```python
from build123d import *

# Parameters (mm, degrees)
SKETCH_1_R                    = 85
EXTRUDE_1_DEPTH               = 50
HOLE_WIZARD_M12_1_D           = 13
HOLE_WIZARD_M12_1_CBORE_D     = 22
HOLE_WIZARD_M12_1_CBORE_DEPTH = 15
PATTERN_CIRCULAR_1_COUNT      = 8
SKETCH_6_W                    = 44.766058572
SKETCH_6_H                    = 9.083836387
SKETCH_6_H_2                  = 8.147377862
CUT_EXTRUDE_1_DEPTH           = 131.192165663
SKETCH_7_R                    = 16
CUT_EXTRUDE_2_DEPTH           = 20
SKETCH_8_R                    = 9
CUT_EXTRUDE_3_DEPTH           = 175.530799574
CHAMFER_1_SIZE                = 2
SKETCH_9_R                    = 55
EXTRUDE_2_DEPTH               = 40
SKETCH_10_R                   = 22.5
CUT_EXTRUDE_4_DEPTH           = 149.489056836
SKETCH_11_W                   = 1.5
SKETCH_11_H                   = 3
CHAMFER_2_SIZE                = 5
CHAMFER_3_SIZE                = 2
CHAMFER_4_SIZE                = 2


with BuildPart() as part:
    # 草圖1 → 填料-伸長1 (new body)
    with BuildSketch(Plane(origin=(0, 0, 0), x_dir=(1, 0, 0), z_dir=(0, 1, 0))):
        with Locations(Location((0, 0, 0), (0, 0, 270))):
            Circle(SKETCH_1_R)
    extrude(amount=EXTRUDE_1_DEPTH)

    # M12 六角頭螺栓的柱孔1 (through all)
    with Locations(Plane.XZ):
        with Locations((-64.671567276, 26.787840266)):
            hole_wizard_m12_1 = CounterBoreHole(HOLE_WIZARD_M12_1_D / 2, HOLE_WIZARD_M12_1_CBORE_D / 2, HOLE_WIZARD_M12_1_CBORE_DEPTH)

    # 環狀複製排列1: M12 六角頭螺栓的柱孔1 ×8 about axis
    pattern_circular_1_axis = Axis((0, 0, 0), (0, 1, 0))
    for i in range(1, PATTERN_CIRCULAR_1_COUNT):
        add(hole_wizard_m12_1.rotate(pattern_circular_1_axis, i * 360 / PATTERN_CIRCULAR_1_COUNT), mode=Mode.SUBTRACT)

    # 草圖6 → 除料-伸長1 (cut, through all)
    with BuildSketch(Plane(origin=(0, 50, 0), x_dir=(1, 0, 0), z_dir=(0, 1, 0))):
        with Locations((0, 86.541918194)):
            Rectangle(SKETCH_6_W, SKETCH_6_H)
        with Locations((0, -86.073688931)):
            Rectangle(SKETCH_6_W, SKETCH_6_H_2)
    extrude(amount=-CUT_EXTRUDE_1_DEPTH, mode=Mode.SUBTRACT)

    # 草圖7 → 除料-伸長2 (cut)
    with BuildSketch(Plane(origin=(0, 0, -82), x_dir=(-1, 0, 0), z_dir=(0, 0, -1))):
        with Locations((0, 30)):
            Circle(SKETCH_7_R)
    cut_extrude_2 = extrude(amount=-CUT_EXTRUDE_2_DEPTH, mode=Mode.SUBTRACT)

    # 鏡射1: 除料-伸長2 across plane
    add(cut_extrude_2.mirror(Plane.XY), mode=Mode.SUBTRACT)

    # 草圖8 → 除料-伸長3 (cut, through all)
    with BuildSketch(Plane.XY.offset(62)):
        with Locations((0, 30)):
            Circle(SKETCH_8_R)
    extrude(amount=-CUT_EXTRUDE_3_DEPTH, mode=Mode.SUBTRACT)

    # 導角1
    chamfer_1_edges = [part.edges().sort_by_distance(p)[0] for p in [
        (-85, 50, 0),
        (-85, 0, 0),
        (85, 50, 0),
        (85, 0, 0),
    ]]
    chamfer(chamfer_1_edges, length=CHAMFER_1_SIZE)

    # 草圖9 → 填料-伸長2 (add)
    with BuildSketch(Plane.XZ):
        with Locations(Location((0, 0, 0), (0, 0, 90))):
            Circle(SKETCH_9_R)
    extrude(amount=EXTRUDE_2_DEPTH)

    # 草圖10 → 除料-伸長4 (cut, through all)
    with BuildSketch(Plane.XZ.offset(40)):
        with Locations(Location((0, 0, 0), (0, 0, 270))):
            Circle(SKETCH_10_R)
    extrude(amount=-CUT_EXTRUDE_4_DEPTH, mode=Mode.SUBTRACT)

    # 草圖11 → 除料-旋轉1 (revolve, cut)
    with BuildSketch(Plane.XY, mode=Mode.PRIVATE) as cut_revolve_1_sk:
        with Locations((-23.25, -25.5)):
            Rectangle(SKETCH_11_W, SKETCH_11_H)
        with Locations((-23.25, -17.5)):
            Rectangle(SKETCH_11_W, SKETCH_11_H)
        with Locations((-23.25, -33.5)):
            Rectangle(SKETCH_11_W, SKETCH_11_H)
        with Locations((-23.25, -9.5)):
            Rectangle(SKETCH_11_W, SKETCH_11_H)
        with Locations((-23.25, -1.5)):
            Rectangle(SKETCH_11_W, SKETCH_11_H)
    revolve(cut_revolve_1_sk.sketch.rotate(Axis((0, -1030.493185966, 0), (0, 1, 0)), 270), axis=Axis((0, -1030.493185966, 0), (0, 1, 0)), mode=Mode.SUBTRACT)

    # 導角2
    chamfer_2_edges = [part.edges().sort_by_distance(p)[0] for p in [
        (0, -40, 22.5),
    ]]
    chamfer(chamfer_2_edges, length=CHAMFER_2_SIZE - 0.0001)  # a hair under: the kernel refuses the full size

    # 導角3
    chamfer_3_edges = [part.edges().sort_by_distance(p)[0] for p in [
        (0, -40, -55),
    ]]
    chamfer(chamfer_3_edges, length=CHAMFER_3_SIZE)

    # 導角4
    chamfer_4_edges = [part.edges().sort_by_distance(p)[0] for p in [
        (0, 50, 22.5),
    ]]
    chamfer(chamfer_4_edges, length=CHAMFER_4_SIZE)


solid = part.part
```
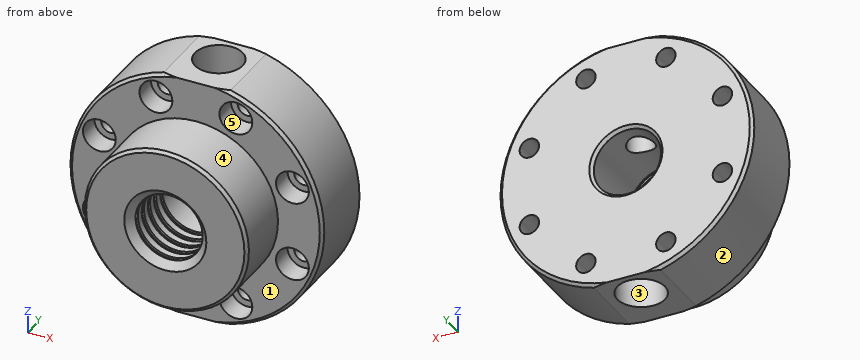
CAD build for the part. Positions are in the model's coordinates, mm. Face numbers are marked on the shaded views. A direction names the side the tool comes from. Round coordinates to 2 decimals unless told otherwise and drop trailing zeros. Answer in a Markdown table with one row per item. Add a question column.
Item 1: Saw through at A-A, the plane y = 30. Count the separate pieces of the cut face and the enclosed holes in it, then the cut area to 3 significant figures.
Item 2: Drill centre lines: line 1 (X direction, y = 4, z = -2); line 2 (Z direction, x = -63, y = 3); line 3 (Y direction, x = 0, z = -69). Where is each one in solid material? Low to high. Write a range as from..to.
Item 3: Drop flat-ended pins along their axis: pin 1 Ø6 at (y, z) = (18.5, 24) entering from -X; pin 2 Ø24 at (x, z) = (69.5, 25) entering from -Y; pin 3 Ø24 at (x, z) = (-6.5, -8.5) entering from -Y; pin 4 Ø8 at (x, z) = (-2.5, -54) entering from -Y. Give the stop position or say it passes through.
Item 4: Which spindle directions (+Z, -Z, +X, -X, +Y, -Y) get a long thin tool onto all of the face, cutting with end or side? Do the marked faces 1 and 2. Say none if no direction does.
Item 5: Mould opens along Z. For the marked faces 3, 4 and 5 say: pulls with the +Z half, pulls with the -Z half, needs draft (parallel to the pull), parting line crosses it, or undercut.
Findings below:
| question | item | result |
|---|---|---|
| 1 | separate pieces | 2 |
| 1 | enclosed holes | 8 |
| 1 | area | 17,100 mm^2 |
| 2 | line 1 | x = -84.98..-22.41, 22.41..84.98 |
| 2 | line 2 | z = -57.06..-37.66, -15.92..15.92, 37.66..57.06 |
| 2 | line 3 | y = 0..14, 46..50 |
| 3 | pin 1 | stops at x = -82.37 |
| 3 | pin 2 | stops at y = 0 |
| 3 | pin 3 | stops at y = -35.2 |
| 3 | pin 4 | stops at y = -40 |
| 4 | face 1 | -Y |
| 4 | face 2 | -X, +Y, -Y |
| 5 | face 3 | needs draft |
| 5 | face 4 | parting line crosses it |
| 5 | face 5 | undercut |
